Autodesk Inventor part; units mm, degrees
ref_plane "YZ Plane" through (0, 0, 0) normal (1, 0, 0) x (0, 1, 0)
ref_plane "XZ Plane" through (0, 0, 0) normal (0, 1, 0) x (-1, 0, 0)
ref_plane "XY Plane" through (0, 0, 0) normal (0, 0, 1) x (1, 0, 0)
ref_plane "작업 평면1" through (0, 0, 0) normal (0, 0, 1) x (1, 0, 0)
sketch "스케치1" plane through (0, 0, 0) normal (0, 0, 1) x (1, 0, 0)
  line L0 (3.5511, -14.2422) -> (3.5511, 14.2422)
  line L1 (-3.5511, 14.2422) -> (-3.5511, -14.2422)
  line L2 (-3.5511, -14.2422) -> (3.5511, -14.2422)
  circle A0 centre (0, 0) radius 13.8
  line L3 (3.5511, 14.2422) -> (-3.5511, 14.2422)
  line L4 (13.8, 0) -> (13.8, 30.0667)
  line L5 (13.8, 30.0667) -> (-13.8, 30.0667)
  line L6 (-13.8, 30.0667) -> (-13.8, 0)
  circle A1 centre (0, 0) radius 13.8
  circle A2 centre (0, 0) radius 7.2
  circle A3 centre (0, -11) radius 1.2812
  circle A4 centre (-7.7782, -7.7782) radius 1.2812
  circle A5 centre (-11, 0) radius 1.2812
  circle A6 centre (-7.7782, 7.7782) radius 1.2812
  circle A7 centre (0, 11) radius 1.2812
  circle A8 centre (7.7782, 7.7782) radius 1.2812
  circle A9 centre (11, 0) radius 1.2812
  circle A10 centre (7.7782, -7.7782) radius 1.2812
  circle A11 centre (11, 27.3) radius 1.35
  circle A12 centre (-11, 27.3) radius 1.35
  point P0 (0, 0)
  point P1 (3.5511, -6.2634)
  point P2 (3.5511, -13.3353)
  point P3 (-3.5511, -13.3353)
  point P4 (-3.5511, -6.2634)
extrude "돌출1" add sketch "스케치1" along normal blind 6 contours L0 A2 A0 | A0 L1 A2 | A0 L0 L3 L1 L6 L5 L4 | A2 L1 A0 L0 | A0 L1 L3 L0 picked at (-2.7821, 10.0973)
properties part number "_thigh_2"
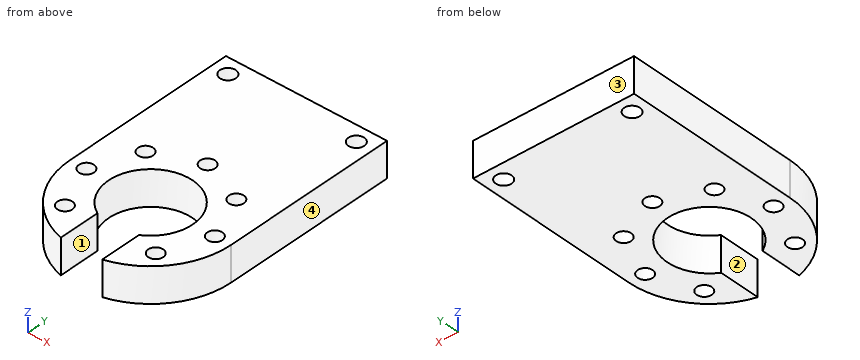
Build history of the part. All positions in model axes, mm. Face numbers are marked on the shaded views. Coordinates: 2 decimals unless noted, no trailing zeros. Order: outer loops, then holes, each group sorted by start corner. A loop starts at its lowest first (then second) coordinate and runs counter-clockwise, first axis right, second up. Notation, with made-up numbers: (10, 49.5) - (57, 49.5) arc R8 cw to (57, 62.5) - close; hole circle Ø6 at (47, 50.25). An arc over 180 degrees is marked (long way). Write item = value, one per line. Start each with the question number.
1) Flat gauge pins, fed straight in: pin 1 Ø2 at (x, y) = (-7.78, -7.78) entering from -Z; pin 2 Ø3 at (x, z) = (5.5, 1) entering from -Y; pin 3 Ø1.8 at (y, z) = (-11, 1.5) entering from -X; pin 4 Ø3 at (y, z) = (-9.5, 2) entering from +X. Where does each tip first touch, or does it go through?
2) Saw through at B-B on x = 0. Write the cut outline in (y, z), then the cut area to 3 significant figures.
3) Two-plate mould, pull along X, no slides. Class the marked faces 1, 2, 3 and 4: pulls with the +X half, pulls with the -X half, needs draft (parallel to the pull), parting line crosses it, or undercut.
4) Saw through at C-C on y = 27.3. Write the cut outline in (x, z).
5) Saw through at A-A on y = 11. Write the cut outline in (x, z).
6) Wall check: line 1 along Y through (x, z) = (-12, 3.3); line 2 along X through (y, z) = (26.5, 4.85); line 3 along Y through (x, z) = (11, 2.1). Give the ranges that are in metal, low to high. Write a range as from..to.
7) Saw through at D-D on z = 3.4. Count the separate pieces of the cut face and the enclosed holes in it, then the cut area to 3 significant figures.
From the geometry:
q1.pin_1 = through
q1.pin_2 = -13.21
q1.pin_3 = -9.4
q1.pin_4 = 11.24
q2.outline = (7.2, 0) - (9.72, 0) - (9.72, 6) - (7.2, 6) - close; (12.28, 0) - (30.07, 0) - (30.07, 6) - (12.28, 6) - close
q2.area = 122 mm^2
q3.face_1 = undercut
q3.face_2 = undercut
q3.face_3 = needs draft
q3.face_4 = pulls with the +X half
q4.outline = (-13.8, 0) - (-12.35, 0) - (-12.35, 6) - (-13.8, 6) - close; (-9.65, 0) - (9.65, 0) - (9.65, 6) - (-9.65, 6) - close; (12.35, 0) - (13.8, 0) - (13.8, 6) - (12.35, 6) - close
q5.outline = (-13.8, 0) - (-1.28, 0) - (-1.28, 6) - (-13.8, 6) - close; (1.28, 0) - (13.8, 0) - (13.8, 6) - (1.28, 6) - close
q6.line_1 = -6.81..-0.8, 0.8..26.39, 28.21..30.07
q6.line_2 = -13.8..-12.09, -9.91..9.91, 12.09..13.8
q6.line_3 = -8.33..-1.28, 1.28..25.95, 28.65..30.07
q7.separate_pieces = 1
q7.enclosed_holes = 9
q7.area = 871 mm^2
